from build123d import *

# Parameters (mm, degrees)
SKETCH15_W                                    = 20
SKETCH15_H                                    = 20
SKETCH15_W_2                                  = 16
SKETCH15_H_2                                  = 16
AL_TUBE_SQUARE_AL_TUBE_0_75_SQR_X_0_065_DEPTH = 988.9
SKETCH16_R                                    = 5
CUT_EXTRUDE1_DEPTH                            = 990.152773842
CUT_EXTRUDE3_DEPTH                            = 990.152773842
CUT_EXTRUDE4_DEPTH                            = 990.152773842
CUT_EXTRUDE4_DEPTH_BACK                       = 990.152773842
SKETCH19_W                                    = 20
SKETCH19_H                                    = 100
BOSS_EXTRUDE1_DEPTH                           = 2
SKETCH20_W                                    = 23.776793386
SKETCH20_H                                    = 100
BOSS_EXTRUDE2_DEPTH                           = 2
SKETCH22_R                                    = 3.125
CUT_EXTRUDE5_DEPTH                            = 2
SKETCH23_R                                    = 3.125
CUT_EXTRUDE6_DEPTH                            = 2


with BuildPart() as part:
    # Sketch15 → Al tube square AL TUBE 0.75 SQR X 0.065 WALL(1) (new body)
    with BuildSketch(Plane(origin=(0, 0, 0), x_dir=(-1, 0, 0), z_dir=(0, 1, 0))):
        Rectangle(SKETCH15_W, SKETCH15_H)
        Rectangle(SKETCH15_W_2, SKETCH15_H_2, mode=Mode.SUBTRACT)
    extrude(amount=AL_TUBE_SQUARE_AL_TUBE_0_75_SQR_X_0_065_DEPTH)

    # Sketch16 → Cut-Extrude1 (cut, through all)
    with BuildSketch(Plane.XY.offset(10)):
        with Locations((0, 10)):
            Circle(SKETCH16_R)
    extrude(amount=-CUT_EXTRUDE1_DEPTH, mode=Mode.SUBTRACT)

    # Sketch17 → Cut-Extrude3 (cut, through all)
    with BuildSketch(Plane.XY.offset(10)):
        Polygon((10, 988.9), (-10, 976.041699033), (-10, 988.9), align=None)
    extrude(amount=-CUT_EXTRUDE3_DEPTH, mode=Mode.SUBTRACT)

    # Sketch18 → Cut-Extrude4 (cut, two sides: drawn at the far end of the back side and taken through both)
    with BuildSketch(Plane(origin=(0, 0, -10), x_dir=(-1, 0, 0), z_dir=(0, 0, -1)).offset(-CUT_EXTRUDE4_DEPTH_BACK)):
        Polygon((-15.481315588, 0.33029398), (41.362305483, 88.745740497), (41.362305483, -42.243020437), (-15.481315588, -42.243020437), align=None)
    extrude(amount=CUT_EXTRUDE4_DEPTH + CUT_EXTRUDE4_DEPTH_BACK, mode=Mode.SUBTRACT)

    # Sketch19 → Boss-Extrude1 (add)
    with BuildSketch(Plane(origin=(11.103958871, 7.138902254, 0), x_dir=(0, 0, 1), z_dir=(-0.8411563188826338, -0.5407920554185471, 0))):
        with Locations((0, 20.532769961)):
            Rectangle(SKETCH19_W, SKETCH19_H)
    extrude(amount=BOSS_EXTRUDE1_DEPTH)

    # Sketch20 → Boss-Extrude2 (add)
    with BuildSketch(Plane(origin=(-446.916807879, 695.141308374, 0), x_dir=(0.8411563188826335, 0.5407920554185475, 0), z_dir=(-0.5407920554185475, 0.8411563188826335, 0))):
        with Locations((531.312430099, 0)):
            Rectangle(SKETCH20_W, SKETCH20_H)
    extrude(amount=BOSS_EXTRUDE2_DEPTH)

    # Sketch22 → Cut-Extrude5 (cut)
    with BuildSketch(Plane(origin=(-447.998391989, 696.823621012, 0), x_dir=(0.8411563188826324, 0.5407920554185492, 0), z_dir=(-0.5407920554185492, 0.8411563188826324, 0))):
        with Locations(Location((531.312430099, 37.5, 0), (0, 0, 180))):
            Circle(SKETCH22_R)
        with Locations(Location((531.312430099, -37.5, 0), (0, 0, 180))):
            Circle(SKETCH22_R)
    extrude(amount=-CUT_EXTRUDE5_DEPTH, mode=Mode.SUBTRACT)

    # Sketch23 → Cut-Extrude6 (cut)
    with BuildSketch(Plane(origin=(11.103958871, 7.138902254, 0), x_dir=(0, 0, -1), z_dir=(0.8411563188826338, 0.540792055418547, 0))):
        with Locations(Location((0, -13.712927992, 0), (0, 0, 90))):
            Circle(SKETCH23_R)
    extrude(amount=-CUT_EXTRUDE6_DEPTH, mode=Mode.SUBTRACT)


solid = part.part
Here's how the part is built. I have some questions about the finished solid (model axes, mm). A direction names the side the tool comes from. Give positions to 0.01 mm unless a question says otherwise; leave off trailing zeros. Loops run counter-clockwise (first coordinate to the right, second up) from the corner with the lowest first, then second, coordinate; pieces in that order, holes last. Notation, with made-up numbers: (81.25, -19) -> (138.25, -19) arc R20 cw to (138.25, 13) -> close; hole circle Ø6 at (67, 66). An arc over 180 degrees is marked (long way). Answer as a JSON object with one key per item and string values. Group by question number.
Item 1: Imagine slicing it at A-A on y = 422. Write out the boundary of the cut face in (x, z).
Item 2: I need wall thicknesses on L1, parallel to X at y = 553, z = 5; L2, parallel to Y at x = -9.5, z = -22. Which ranges of each line are inside material? Lowest first, please.
Item 3: Will these pins go through, and if not, where does the flat tip stop? pin 1 (1.5 mm diameter, centred on x = -17.5, z = 8.5, fed in from -Y); pin 2 (13 mm diameter, centred on y = 594.5, z = 4, fed in from -X); pin 3 (17.5 mm diameter, centred on y = 501.5, z = 1, fed in from +X).
Item 4: On a 3-axis mill with a long thin cutter (end or side, diameter ignored), from which of +Z, -Z, +X, -X, +Y, -Y can I reach the whole of each face in a straight line? I mean faces 1 (the flat face through (-0.11, 24.58, -0.11)), 2 (the flat face through (-0.14, 982.38, -30.28)), 3 (the flat face through (-0.14, 982.38, 29.72)), 4 (the flat face through (10, 492, 0)). Say none if no direction works.
Item 5: Imagine slicing it at B-B on z = -22.5. Write out the boundary of the cut face in (x, y), then the cut area to 3 significant figures.
Item 6: Thinking about a two-plate mould opening in Y: for faces 5 (the flat face through (-2.061, 23.917, -0.14)), 6 (the flat face through (16.51, -1.27, -0.14)), 7 (the flat face through (4, 436, 10)), 8 (the flat face through (-0.11, 982.4, -0.11)), which applies, pulls with the +Y half, pulls with the -Y half, needs draft (parallel to the pull), parting line crosses it, or undercut?
Answer list:
{
 "1": {"outline": "(-10, -10) -> (10, -10) -> (10, 10) -> (-10, 10) -> close; hole (-8, -8) -> (8, -8) -> (8, 8) -> (-8, 8) -> close"},
 "2": {"L1": "x = -10 to -8, 8 to 10", "L2": "y = 976.36 to 978.74"},
 "3": {"pin 1": "stops at y = 46.77", "pin 2": "stops at x = -10", "pin 3": "stops at x = 10"},
 "4": {"face 1": "none", "face 2": "-Z, +X, -Y", "face 3": "+Z, +X, -Y", "face 4": "+Z, -Z, +X, +Y"},
 "5": {"outline": "(-11.08, 977.72) -> (-10, 976.04) -> (10, 988.9) -> (8.92, 990.58) -> close", "area": "47.6 mm2"},
 "6": {"face 5": "pulls with the -Y half", "face 6": "pulls with the +Y half", "face 7": "needs draft", "face 8": "undercut"}
}
